Verification items for the finished model (mm, model axes). A direction names the side the tool comes from. Round coordinates to 2 decimals unless told otherwise and drop trailing zeros. Order: outer loops, then holes, each group sorted by start corner. A loop starts at its lowest first (then second) coordinate and runs counter-clockwise, first axis right, second up.
```python
from build123d import *

# Parameters (mm, degrees)
SKETCH1_W           = 92
SKETCH1_H           = 6
BOSS_EXTRUDE1_DEPTH = 50
SKETCH2_W           = 6
SKETCH2_H           = 6
BOSS_EXTRUDE2_DEPTH = 6
SKETCH3_R           = 6
CUT_EXTRUDE1_DEPTH  = 6


with BuildPart() as part:
    # Sketch1 → Boss-Extrude1 (new body)
    with BuildSketch(Plane.XY):
        with Locations((0, 3)):
            Rectangle(SKETCH1_W, SKETCH1_H)
    extrude(amount=BOSS_EXTRUDE1_DEPTH)

    # Sketch2 → Boss-Extrude2 (add)
    with BuildSketch(Plane(origin=(0, 0, 0), x_dir=(-1, 0, 0), z_dir=(0, 0, -1))):
        with Locations((-33, 3)):
            Rectangle(SKETCH2_W, SKETCH2_H)
        with Locations((33, 3)):
            Rectangle(SKETCH2_W, SKETCH2_H)
    extrude(amount=BOSS_EXTRUDE2_DEPTH)

    # Sketch3 → Cut-Extrude1 (cut)
    with BuildSketch(Plane.XZ):
        with Locations((21, 9)):
            Circle(SKETCH3_R)
    extrude(amount=-CUT_EXTRUDE1_DEPTH, mode=Mode.SUBTRACT)


solid = part.part
```
1) Sectioned sample at C-C on y = 2.4. Record the cut outline in (x, z), then the cut area to 3 significant figures.
2) Scan lines: probe 1 along Z at (x, y) = (21, 3); probe 2 along Z at (x, y) = (-40.5, 1.4); probe 3 along X at (y, z) = (0.5, 10). Record each from-to range of solid material in increasing order.
3) Go/stop test with flat-tipped pins: pin 1 Ø7 at (x, z) = (21, 9) entering from +Y; pin 2 Ø1.8 at (x, y) = (1.5, 4.5) entering from -Z. Record where each tip stops, or that it passes through.
4) Sectioned sample at A-A on z = -2. Record the cut outline in (x, y).
5) Tool access check on faces 1 (the flat face through (-33, 3, -6)), 2 (the flat face through (36, 3, -3)), 3 (the flat face through (-30, 3, -3)), 4 (the flat face through (-41, 3, 0)). Record the directions out of +Z, -Z, +X, -X, +Y, -Y that give a thin tool (end or side, any length) a straight path to the whole face; none if there is none.
6) Draft check along X on faces 5 (the flat face through (30, 3, -3)), 6 (the flat face through (-1, 3, 50)), 7 (the flat face through (-46, 3, 25)). Enter one of: released by +X, released by -X, zero draft, split by the parting line, or undercut.
7) Sectioned sample at B-B on x = 21. Record the cut outline in (y, z).
Returned:
1. outline: (-46, 0) - (-36, 0) - (-36, -6) - (-30, -6) - (-30, 0) - (30, 0) - (30, -6) - (36, -6) - (36, 0) - (46, 0) - (46, 50) - (-46, 50) - close; hole circle Ø12 at (21, 9)
1. area: 4,560 mm2
2. probe 1: z = 0 to 3, 15 to 50
2. probe 2: z = 0 to 50
2. probe 3: x = -46 to 15.08, 26.92 to 46
3. pin 1: passes through
3. pin 2: stops at z = 0
4. outline: (-36, 0) - (-30, 0) - (-30, 6) - (-36, 6) - close; (30, 0) - (36, 0) - (36, 6) - (30, 6) - close
5. face 1: -Z, +X, -X, +Y, -Y
5. face 2: -Z, +X, +Y, -Y
5. face 3: -Z, +Y, -Y
5. face 4: -Z, -X, +Y, -Y
6. face 5: undercut
6. face 6: zero draft
6. face 7: released by -X
7. outline: (0, 0) - (6, 0) - (6, 3) - (0, 3) - close; (0, 15) - (6, 15) - (6, 50) - (0, 50) - close
